Source: CAD feature listing. Evaluate the final solid. Frame: model axes, mm. A direction names the side the tool comes from. Give positions to 0.01 mm unless a question says otherwise; leave off trailing zeros. Order: outer loops, then holes, each group sorted by start corner. A loop starts at its lowest first (then second) coordinate and runs counter-clockwise, first axis right, second up.
Autodesk Fusion 360 part; units mm, degrees
sketch "Skizze1" plane through (0, 0, 0) normal (0, 0, 1) x (1, 0, 0)
  line L0 (19.5, 14) -> (-19.5, 14)
  line L1 (-19.5, 14) -> (-19.5, -14)
  line L2 (-19.5, -14) -> (19.5, -14)
  line L3 (19.5, -14) -> (19.5, 14)
  line L4 (19.5, 14) -> (-19.5, -14) construction
  line L5 (-19.5, 14) -> (19.5, -14) construction
  line L6 (22.5, 17) -> (-22.5, 17)
  line L7 (-22.5, 17) -> (-22.5, -17)
  line L8 (-22.5, -17) -> (22.5, -17)
  line L9 (22.5, -17) -> (22.5, 17)
  line L10 (22.5, 17) -> (-22.5, -17) construction
  line L11 (-22.5, 17) -> (22.5, -17) construction
  line L12 (15.5, 14) -> (-15.5, 14)
  line L13 (-15.5, 14) -> (-15.5, -14)
  line L14 (-15.5, -14) -> (15.5, -14)
  line L15 (15.5, -14) -> (15.5, 14)
  line L16 (15.5, 14) -> (-15.5, -14) construction
  line L17 (-15.5, 14) -> (15.5, -14) construction
  line L18 (-19.5, 14) -> (-18.5, 14)
  circle A0 centre (-18, 12) radius 1
  circle A1 centre (-18, -12) radius 1
  circle A2 centre (18, -12) radius 1
  circle A3 centre (18, 12) radius 1
  dimension "d1" = 39
  dimension "d2" = 28
  dimension "d3" = 45
  dimension "d4" = 34
  dimension "d5" = 31
  dimension "d7" = 2
  dimension "d8" = 2
  dimension "d9" = 2
  dimension "d10" = 2
extrude "Extrusion1" add sketch "Skizze1" along normal blind 6 contours L6 L7 L8 L9
extrude "Extrusion2" add sketch "Skizze1" along normal blind 2 contours L0 L2 L3 L15 | L0 L1 L2 L13 L18
extrude "Extrusion3" add 1 faces at (-6.5, -16, 6) along direction (0, 0, 1) blind 2
extrude "Extrusion4" add 1 faces at (-22.5, -5.6667, 5.3333) along direction (-1, 0, 0) blind 2
extrude "Extrusion5" add 1 faces at (22.5, -5.6667, 2.6667) along direction (1, 0, 0) blind 2
extrude "Extrusion6" add 1 faces at (-8.1667, -17, 5.3333) along direction (0, -1, 0) blind 2
extrude "Extrusion7" add 1 faces at (8.1667, 17, 5.3333) along direction (0, 1, 0) blind 2
fillet "Abrundung1" radius 4 1 edges at (24.5, 19, 4)
fillet "Abrundung2" radius 4 1 edges at (-24.5, 19, 4)
fillet "Abrundung3" radius 4 1 edges at (-24.5, -19, 4)
fillet "Abrundung4" radius 4 1 edges at (24.5, -19, 4)
chamfer "Fase1" distance 2 angle 45 8 edges at (24.5, 0, 0) (23.3284, -17.8284, 0) (0, -19, 0) (-23.3284, -17.8284, 0) (-24.5, 0, 0) (-23.3284, 17.8284, 0) (0, 19, 0) (23.3284, 17.8284, 0)
sketch "Skizze2" plane through (24.5, 0, 0) normal (1, 0, 0) x (0, 0, -1)
  line L0 (-2, -15) -> (-2, 15)
  line L1 (-2, 15) -> (-8, 15)
  line L2 (-8, 15) -> (-8, -15)
  line L3 (-8, -15) -> (-2, -15)
  line L4 (-7, 15) -> (-4.5, 15)
  line L5 (-4.5, 15) -> (-4.5, -15)
  line L6 (-4.5, -15) -> (-7, -15)
  line L7 (-7, -15) -> (-7, 15)
extrude "Extrusion8" cut sketch "Skizze2" against normal blind 44 contours L1 L3 L4 L5 L6 L7
sketch "Skizze3" plane through (0, 0, 0) normal (1, 0, 0) x (0, 0, -1)
  line L0 (-4.5, -14) -> (-2, -14)
  line L1 (-2, -14) -> (-2, 14)
  line L2 (-2, 14) -> (-4.5, 14)
  line L3 (-4.5, 14) -> (-4.5, 15)
  line L4 (-4.5, 15) -> (-7, 15)
  line L5 (-7, 15) -> (-7, 14)
  line L6 (-7, 14) -> (-8, 14)
  line L7 (-8, 14) -> (-8, -14)
  line L8 (-8, -14) -> (-7, -14)
  line L9 (-7, -14) -> (-7, -15)
  line L10 (-7, -15) -> (-4.5, -15)
  line L11 (-4.5, -15) -> (-4.5, -14)
  line L12 (-7, 15) -> (-4.5, 15)
  line L13 (-4.5, 15) -> (-4.5, 11)
  line L14 (-4.5, 11) -> (-7, 11)
  line L15 (-7, 11) -> (-7, 15)
  line L16 (-7, -15) -> (-4.5, -15)
  line L17 (-4.5, -15) -> (-4.5, -11)
  line L18 (-4.5, -11) -> (-7, -11)
  line L19 (-7, -11) -> (-7, -15)
  dimension "d37" = 4
  dimension "d38" = 2.5
  dimension "d39" = 4
  dimension "d40" = 2.5
extrude "Extrusion9" cut sketch "Skizze3" against normal blind 21 contours L9 L10 L11 L16 L17 L18 L19 | L3 L4 L5 L12 L13 L14 L15
sketch "Skizze4" plane through (19.5, 0, 0) normal (-1, 0, 0) x (0, 0, 1)
  line L0 (7, 14) -> (7, -14)
  line L1 (7, -14) -> (8, -14)
  line L2 (8, -14) -> (8, 14)
  line L3 (8, 14) -> (7, 14)
  line L4 (7, 14) -> (8, 14)
  line L5 (8, 14) -> (8, -14)
  line L6 (8, -14) -> (7, -14)
  line L7 (7, -14) -> (7, 14)
extrude "Extrusion10" cut sketch "Skizze4" against normal blind 5
1) Section query C-C, the plane x = 6. Return the cut outline in (y, z), and give its area (3 significant figures).
Report:
outline: (-19, 2) - (-17, 0) - (-14, 0) - (-14, 4.5) - (-15, 4.5) - (-15, 7) - (-14, 7) - (-14, 8) - (-19, 8) - close; (14, 0) - (17, 0) - (19, 2) - (19, 8) - (14, 8) - (14, 7) - (15, 7) - (15, 4.5) - (14, 4.5) - close
area: 71.0 mm2
2) Draft query along Y for faces 1 (the flat face through (0, 18, 1)), 2 (the cylindrical face through (23.359, -17.797, 4.958)), 3 (the flat face through (0.2, -14.2, 7)). Return one class per face: +Y half, -Y half, draft (parallel to the pull), parting line (faces both ways), or undercut.
Report:
face 1: +Y half
face 2: -Y half
face 3: undercut
3) Section query B-B, the plane y = -9. Return the cut outline in (x, z).
Report:
outline: (-24.5, 2) - (-22.5, 0) - (-15.5, 0) - (-15.5, 2) - (-19.5, 2) - (-19.5, 8) - (-24.5, 8) - close; (15.5, 0) - (22.5, 0) - (24.5, 2) - (24.5, 4.5) - (19.5, 4.5) - (19.5, 2) - (15.5, 2) - close
4) Section query A-A, the plane x = 18. Return the cut outline in (y, z), and give its area (3 significant figures).
Report:
outline: (-19, 2) - (-17, 0) - (-13, 0) - (-13, 2) - (-14, 2) - (-14, 4.5) - (-15, 4.5) - (-15, 7) - (-14, 7) - (-14, 8) - (-19, 8) - close; (-11, 0) - (11, 0) - (11, 2) - (-11, 2) - close; (13, 0) - (17, 0) - (19, 2) - (19, 8) - (14, 8) - (14, 7) - (15, 7) - (15, 4.5) - (14, 4.5) - (14, 2) - (13, 2) - close
area: 119 mm2
5) Material intervals for L1, parallel to X at y = 6, z = 3; L2, parallel to Y at x = 18, z = 0.5; L3, parallel to Y at x = -18, z = 1.3, sorted ascending.
Report:
L1: x = -24.5 to -19.5, 19.5 to 24.5
L2: y = -17.5 to -13, -11 to 11, 13 to 17.5
L3: y = -18.3 to -13, -11 to 11, 13 to 18.3
6) Pin query (flat end, axial travel): pin 1 (1 mm diameter, centred on x = 19.5, z = 1, fed in from +Y); pin 2 (0.6 mm diameter, centred on y = 6, z = 1, fed in from +X); pin 3 (3 mm diameter, centred on y = 12.5, z = 5.5, fed in from +X); pin 4 (2 mm diameter, centred on x = 17, y = 4.5, fed in from +Z). Return the tip coordinate at first contact, or that it passes through.
Report:
pin 1: stops at y = 18.5
pin 2: stops at x = 23.8
pin 3: stops at x = 24.5
pin 4: stops at z = 2
7) Reachability of faces 4 (the flat face through (-20, 11, 6)), 5 (the flat face through (0, 14, 2)), 6 (the flat face through (0, -18, 1)), 7 (the flat face through (2.2, 14, 7.5)) from +Z, -Z, +X, -X, +Y, -Y: full face, straight path, thin tool, end or side. Return the list, or none.
Report:
face 4: +X
face 5: +Z
face 6: -Z, +X, -X, -Y
face 7: +Z, +X
8) Section query D-D, the plane y = 12. Return the cut outline in (x, z).
Report:
outline: (-24.5, 2) - (-22.5, 0) - (-19, 0) - (-19, 2) - (-19.5, 2) - (-19.5, 4.5) - (-21, 4.5) - (-21, 7) - (-19.5, 7) - (-19.5, 8) - (-24.5, 8) - close; (-17, 0) - (-15.5, 0) - (-15.5, 2) - (-17, 2) - close; (15.5, 0) - (17, 0) - (17, 2) - (15.5, 2) - close; (19, 0) - (22.5, 0) - (24.5, 2) - (24.5, 4.5) - (19.5, 4.5) - (19.5, 2) - (19, 2) - close
